The model under review builds one solid part; all positions refer to its coordinate system, in mm. A direction names the side the tool comes from. Give positions to 0.01 mm unless a question says otherwise; leave off trailing zeros. Loops run counter-clockwise (first coordinate to the right, second up) from the corner with the lowest first, then second, coordinate; pieces in that order, holes last. Notation, with made-up numbers: (-31, -30) - (2, -30) arc R23 cw to (2, 0) - close; hole circle Ø9 at (51.25, -18). An arc over 180 degrees is marked (long way). Answer as a JSON object with one key per item and string values.
from build123d import *

# Parameters (mm, degrees)
BOSS_EXTRU_1_DEPTH      = 60
ESQUISSE2_R             = 30
ESQUISSE2_R_2           = 29
BOSS_EXTRU_2_DEPTH      = 60
ESQUISSE3_R             = 25
ENL_V_MAT_EXTRU_1_DEPTH = 27
ESQUISSE5_W             = 17
ESQUISSE5_H             = 21.625890028
ENL_V_MAT_EXTRU_2_DEPTH = 8
ESQUISSE6_R             = 2.225
ENL_V_MAT_EXTRU_3_DEPTH = 2


with BuildPart() as part:
    # Esquisse1 → Boss.-Extru.1 (new body)
    with BuildSketch(Plane.XY):
        with BuildLine():
            Line((1, -15.006468588), (1, -3.354101966))
            ThreePointArc((1, -3.354101966), (3.5, 0), (1, 3.354101966))
            Line((1, 3.354101966), (1, 30))
            Line((1, 30), (-1, 30))
            Line((-1, 30), (-1, 3.354101966))
            ThreePointArc((-1, 3.354101966), (-3.5, 0), (-1, -3.354101966))
            Line((-1, -3.354101966), (-1, -30))
            Line((-1, -30), (1, -30))
            Line((1, -30), (1, -15.006468588))
        make_face()
    extrude(amount=BOSS_EXTRU_1_DEPTH)

    # Esquisse2 → Boss.-Extru.2 (add)
    with BuildSketch(Plane.XY.offset(60)):
        Circle(ESQUISSE2_R)
        Circle(ESQUISSE2_R_2, mode=Mode.SUBTRACT)
    extrude(amount=-BOSS_EXTRU_2_DEPTH)

    # Esquisse3 → Enlèv. mat.-Extru.1 (cut)
    with BuildSketch(Plane.XY.offset(60)):
        Circle(ESQUISSE3_R)
    extrude(amount=-ENL_V_MAT_EXTRU_1_DEPTH, mode=Mode.SUBTRACT)

    # Esquisse5 → Enlèv. mat.-Extru.2 (cut)
    with BuildSketch(Plane.ZY.offset(1)):
        with Locations((24.5, -14.16704698)):
            Rectangle(ESQUISSE5_W, ESQUISSE5_H)
        with Locations((24.5, 14.16704698)):
            Rectangle(ESQUISSE5_W, ESQUISSE5_H)
    extrude(amount=-ENL_V_MAT_EXTRU_2_DEPTH, mode=Mode.SUBTRACT)

    # Esquisse6 → Enlèv. mat.-Extru.3 (cut)
    with BuildSketch(Plane.XY.offset(33)):
        Circle(ESQUISSE6_R)
    extrude(amount=-ENL_V_MAT_EXTRU_3_DEPTH, mode=Mode.SUBTRACT)


solid = part.part
Q1. Clearance check with flat-ended pins moving along their axes: pin 1 Ø0.6 at (x, y) = (-0.5, 14) entering from +Z; pin 2 Ø1.5 at (y, z) = (-3.5, 8) entering from +X; pin 3 Ø3.5 at (x, y) = (1, 0.5) entering from +Z. State where each tip first meets the part, or that it passes through.
Results:
{"pin 1": "stops at z = 16", "pin 2": "stops at x = 29.87", "pin 3": "stops at z = 33"}
Q2. Consider section B-B, the plane y = 0. State the section outline as (x, z) points (3 decimals).
Results:
{"outline": "(-30, 0) - (-29, 0) - (-29, 60) - (-30, 60) - close; (-3.5, 0) - (3.5, 0) - (3.5, 33) - (2.225, 33) - (2.225, 31) - (-2.225, 31) - (-2.225, 33) - (-3.5, 33) - close; (29, 0) - (30, 0) - (30, 60) - (29, 60) - close"}
Q3. For faces 1 (the face through (0, -3.354, 24)), 2 (the face through (-1, 19, 14)), 3 (the face through (0, 30, 30)), list the 3-axis set-ups (+Z, -Z, +X, -X, +Y, -Y) from which the entire face can be reached by the end or side of a thin tool; tool diameter is ignored.
Results:
{"face 1": "+Z", "face 2": "+Z, -Z", "face 3": "+Z, -Z, +X, -X, +Y"}
Q4. To check wall thickness, follow probe 1 along Y at (x, z) = (0, 32.2) (3 decimals); probe 2 along X at (y, z) = (12, 9); probe 3 along X at (y, z) = (-1, 39). State the ranges of each line that lie inside material, in increasing order. Write a range as [from, to].
Results:
{"probe 1": "y = [-30, -24.98], [-3.354, -2.225], [2.225, 3.354], [24.98, 30]", "probe 2": "x = [-27.5, -26.4], [-1, 1], [26.4, 27.5]", "probe 3": "x = [-29.98, -28.98], [28.98, 29.98]"}
Q5. Consider section C-C, the plane x = -17.5. State the section outline as (y, z) points, plus the area to 3 significant figures.
Results:
{"outline": "(-24.37, 0) - (-23.12, 0) - (-23.12, 60) - (-24.37, 60) - close; (23.12, 0) - (24.37, 0) - (24.37, 60) - (23.12, 60) - close", "area": "149 mm^2"}
Q6. Consider section A-A, the plane z = 25.5. State how many separate pieces and enclosed holes the cut face has, plus the area to 3 significant figures.
Results:
{"separate pieces": "2", "enclosed holes": "1", "area": "240 mm^2"}
Q7. The part is to be moulded in two halves that separate along Y. For faces 4 (the face through (3.5, -0.1, 16.3)), 5 (the face through (-28.993, 0.624, 30.42)), 6 (the face through (0, -30, 30)), 7 (the face through (29.993, -0.646, 30.42)), say which applies: +Y half, -Y half, draft (parallel to the pull), parting line (faces both ways), or undercut.
Results:
{"face 4": "undercut", "face 5": "undercut", "face 6": "-Y half", "face 7": "parting line"}
